For this review, take the finished solid that the model builds, in its own axes (mm). A direction names the side the tool comes from. Give positions to 0.01 mm unless a question says otherwise; leave off trailing zeros. Order: outer loops, then holes, each group sorted by start corner. A loop starts at its lowest first (then second) coordinate and runs counter-clockwise, first axis right, second up. Notation, with made-up numbers: M -22.5,79.25 L -6.5,79.25 A32 cw -6.5,108.25 Z; hole C -36,6 d10. An arc over 180 degrees is marked long. Use CSV: the item, a comma, the result in double quotes. Start each with the question number.
(1) Draft analysis for pull direction Z (two halves, no side actions). For faces 4 (the face through (1.52, 18.39, -0.33)), 5 (the face through (1.48, 11.28, -4.85)), 6 (the face through (1, 13, -48)), state which applies: pulls with the +Z half, pulls with the -Z half, needs draft (parallel to the pull), parting line crosses it, or undercut.
(2) Consider section B-B (z = -26.5). Write out the cut boundary in (x, y), and give its area (3 significant figures).
(3) Consider section D-D (z = -18). Write out the cut boundary in (x, y), and give its area (3 significant figures).
(4) Consider section C-C (x = -4). Write out the cut boundary in (y, z), and give its area (3 significant figures).
(5) Tool access review of faces 1 (the face through (0, 14, -9)), 2 (the face through (-5.5, 8, -24)), 3 (the face through (0, 14, -39)): name each direction out of +Z, -Z, +X, -X, +Y, -Y from which nothing blocks a thin tool from reaching the whole face with its end or side.
(6) Consider section A-A (y = 16.5). Write out the cut boundary in (x, z).
(7) Clearance check with flat-ended pins moving along their axes: P1, Ø7, axis at y = 19.5, z = -7.5, coming from the -X side; P2, Ø1, axis at x = -1, z = -22, coming from the +Y side; P3, Ø4.5, axis at y = 13.5, z = -6, coming from the +X side; P4, Ø6, axis at x = -6.5, z = -12, coming from the +Y side. State where each tip first meets the part, or that it passes through.
(8) Wall thickness on L1, parallel to X at y = 23, z = -24.5; L2, parallel to Z at x = -4, y = 15.5; L3, parallel to X at y = 20, z = -3: over which ranges is each line inside the solid? List them lowest first. Write a range as from..to.
```python
from build123d import *

# Parameters (mm, degrees)
SKETCH_1_W          = 48
SKETCH_1_H          = 27
EXTRUDE_1_DEPTH     = 3
SKETCH_5_R          = 13.5
EXTRUDE_2_DEPTH     = 5.5
SKETCH_6_R          = 5
EXTRUDE_3_DEPTH     = 4.5
SKETCH_7_R          = 4
CUT_EXTRUDE_1_DEPTH = 57.586217403
SKETCH_8_R          = 2.5
CUT_EXTRUDE_2_DEPTH = 56.973207877
CUT_EXTRUDE_3_DEPTH = 56.973207877
FILLET_1_R          = 3


with BuildPart() as part:
    # 草图1 → 凸台-拉伸1 (new body)
    with BuildSketch(Plane(origin=(0, 0, 0), x_dir=(0, 0, -1), z_dir=(1, 0, 0))):
        with Locations((24, 13.5)):
            Rectangle(SKETCH_1_W, SKETCH_1_H)
    extrude(amount=EXTRUDE_1_DEPTH)

    # 草图5 → 凸台-拉伸2 (add)
    with BuildSketch(Plane.ZY):
        with Locations(Location((-24, 13.5, 0), (0, 0, 270))):
            Circle(SKETCH_5_R)
    extrude(amount=EXTRUDE_2_DEPTH)

    # 草图6 → 凸台-拉伸3 (add)
    with BuildSketch(Plane.ZY.offset(5.5)):
        with Locations((-24, 13.5)):
            Circle(SKETCH_6_R)
    extrude(amount=EXTRUDE_3_DEPTH)

    # 草图7 → 切除-拉伸1 (cut, through all)
    with BuildSketch(Plane.ZY.offset(10)):
        with Locations((-24, 13.5)):
            Circle(SKETCH_7_R)
    extrude(amount=-CUT_EXTRUDE_1_DEPTH, mode=Mode.SUBTRACT)

    # 草图8 → 切除-拉伸2 (cut, through all)
    with BuildSketch(Plane.ZY):
        with Locations((-42, 13.5)):
            Circle(SKETCH_8_R)
        with Locations((-6, 13.5)):
            Circle(SKETCH_8_R)
    extrude(amount=-CUT_EXTRUDE_2_DEPTH, mode=Mode.SUBTRACT)

    # 草图9 → 切除-拉伸3 (cut, through all)
    with BuildSketch(Plane.ZY):
        Polygon((-36, 27), (-48, 18.580800232), (-48, 27), align=None)
        Polygon((-12, 27), (0, 18.580800232), (0, 27), align=None)
        Polygon((0, 0), (-12, 0), (0, 8.106535138), align=None)
        Polygon((-48, 0), (-48, 8.106535138), (-36, 0), align=None)
    extrude(amount=-CUT_EXTRUDE_3_DEPTH, mode=Mode.SUBTRACT)

    # 圆角1
    fillet_1_edges = [part.edges().sort_by_distance(p)[0] for p in [
        (1.5, 27, -36),
        (1.5, 18.580800232, -48),
        (1.5, 27, -12),
        (1.5, 18.580800232, 0),
        (1.5, 8.106535138, 0),
        (1.5, 0, -12),
        (1.5, 0, -36),
        (1.5, 8.106535138, -48),
    ]]
    fillet(fillet_1_edges, radius=FILLET_1_R)


solid = part.part
```
Check result:
1,face 4,"pulls with the +Z half"
1,face 5,"undercut"
1,face 6,"pulls with the -Z half"
2,outline,"M -10,9.17 L -5.5,9.17 L -5.5,0.23 L 0,0.23 L 0,0 L 3,0 L 3,10.38 L -10,10.38 Z; M -10,16.62 L 3,16.62 L 3,27 L 0,27 L 0,26.77 L -5.5,26.77 L -5.5,17.83 L -10,17.83 Z"
2,area,"185 mm^2"
3,outline,"M -5.5,1.41 L 0,1.41 L 0,0 L 3,0 L 3,27 L 0,27 L 0,25.59 L -5.5,25.59 Z"
3,area,"214 mm^2"
4,outline,"C 13.5,-24 d27; hole C 13.5,-24 d8"
4,area,"522 mm^2"
5,face 1,"+Z, -X"
5,face 2,"-X"
5,face 3,"-Z, -X"
6,outline,"M -10,-28 L -5.5,-28 L -5.5,-37.16 L 0,-37.16 L 0,-48 L 3,-48 L 3,-26.65 L -10,-26.65 Z; M -10,-21.35 L 3,-21.35 L 3,0 L 0,0 L 0,-10.84 L -5.5,-10.84 L -5.5,-20 L -10,-20 Z"
7,P1,"stops at x = 0"
7,P2,"stops at y = 26.92"
7,P3,"passes through"
7,P4,"stops at y = 23.41"
8,L1,"x = -5.5..3"
8,L2,"z = -37.35..-27.46, -20.54..-10.65"
8,L3,"x = 0..3"
